from build123d import *

# Parameters (mm, degrees)
F0_W = 2
F0_H = 9.95


with BuildPart() as f1:
    # F0 (on Front) → F1 (revolve)
    with BuildSketch(Plane.XZ):
        with Locations((0, 65.025)):
            Rectangle(F0_W, F0_H)
    revolve(axis=Axis((8.224491, 0, 0), (1, 0, 0)))

    # F2 (on Front) → F3 (revolve)
    with BuildSketch(Plane.XZ):
        Polygon((-2.720465, 65), (-10, 65), (-10, 60), (-1, 60), (-1, 65), (-8, 70), (-8, 68.771096), align=None)
        Polygon((8.279535, 65), (1, 65), (1, 60), (10, 60), (10, 65), (3, 70), (3, 68.771096), align=None)
    revolve(axis=Axis((3.221242, 0, 0), (1, 0, 0)))


solid = f1.part
Verification items for the finished model (mm, model axes). A direction names the side the tool comes from. Coordinates: 2 decimals unless noted, no trailing zeros.
1. Go/stop test with flat-tipped pins: pin 1 Ø10 at (x, y) = (0.5, 44) entering from -Z; pin 2 Ø10 at (x, y) = (-1.5, 12.5) entering from +Z; pin 3 Ø5 at (x, y) = (1, -19) entering from -Z. Record where each tip stops, or that it passes through.
Results found:
pin 1: stops at z = -58.13
pin 2: stops at z = 69.59
pin 3: stops at z = -68.03
2. Scan lines: line 1 (Z direction, x = 5.25, y = 16); line 2 (Y direction, x = -3, z = 18.5); line 3 (Z direction, x = 5.5, y = 0). Record each from-to range of solid material in increasing order.
Results found:
line 1: z = -66.49 to -65.23, -63 to -57.83, 57.83 to 63, 65.23 to 66.49
line 2: y = -63.8 to -62.52, -62.31 to -57.08, 57.08 to 62.31, 62.52 to 63.8
line 3: z = -68.21 to -66.99, -65 to -60, 60 to 65, 66.99 to 68.21
3. Release check for a two-part mould opening along X. For faces 1 (the face through (-10, 57.5, 19)), 2 (the face through (3, 52, 46)), 3 (the face through (9.56, 63.76, -14.16)) record: +X half, -X half, draft (parallel to the pull), parting line (faces both ways), or undercut.
Results found:
face 1: -X half
face 2: undercut
face 3: +X half
4. Set-up check for faces 4 (the face through (10, 57.5, -19)), 5 (the face through (-1, 46.3, -46.3)), 6 (the face through (-8, 52, 46)): record each of +Z, -Z, +X, -X, +Y, -Y from which the full face is reachable in a straight line by a thin tool's end or side.
Results found:
face 4: +Z, -Z, +X, +Y, -Y
face 5: none
face 6: -X
